The listing builds one solid part. Answer for the finished solid, in the listing's coordinates (mm). Face numbers are marked on the shaded views. Give positions to 0.01 mm unless a question says otherwise; leave off trailing zeros. Order: outer loops, then holes, each group sorted by start corner. A loop starts at its lowest first (then second) coordinate and runs counter-clockwise, first axis right, second up. Notation, with made-up numbers: (-3.5, 72) - (4.5, 72) arc R30 cw to (4.5, 103) - close; hole circle Ø1 at (5, 73). An arc over 180 degrees is marked (long way). Answer as a JSON object with one key per item and string values. Group by question number.
Q1. Given pin 1 (10 mm diameter, centred on x = 122, y = 17, fed in from -Z); pin 2 (1.5 mm diameter, centred on x = 75.5, y = 19, fed in from +Z); pin 3 (12 mm diameter, centred on x = 103, y = -7, fed in from +Z), each flat-ended and moving along its own axis, determine where each tip first touches the part or whether it passes through.
Q2. A cutting plane is placed at A-A, the plane z = -9.5. Give the vertices of the cut face in (x, y), and give its area (3 significant figures).
Q3. A cutting plane is placed at C-C, the plane x = 64. Give the vertices of the cut face in (y, z).
Q4. The mould has two halves that part along Y. Classify the marked faces 1, 2 and 3: released by +Y, released by -Y, zero draft, split by the parting line, or undercut.
Q5. A cutting plane is placed at D-D, the plane z = 49. Give the vertices of the cut face in (x, y), and give its area (3 significant figures).
Q6. Consider line 1 (Z direction, x = 0, y = -1); line 2 (X direction, y = -43, z = 0); line 3 (Y direction, x = 173, z = -2). Determine where each line is inside the solid, lowest interval first.
Q7. A cutting plane is placed at B-B, the plane y = -56.5. Give the vertices of the cut face in (x, z), and give its area (3 significant figures).
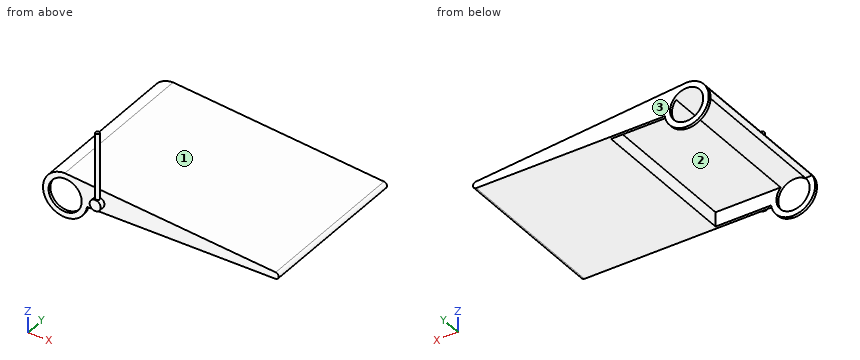
from build123d import *

# Parameters (mm, degrees)
F0_R     = 15
F1_DEPTH = 72.5
F2_W     = 140
F2_H     = 31.716244
F3_DEPTH = 70
F4_R     = 5
F5_DEPTH = 5
F6_R     = 1.75
F7_DEPTH = 70


with BuildPart() as f1:
    # F0 (on Front) → F1 (new body, symmetric)
    with BuildSketch(Plane.XZ):
        with BuildLine():
            Line((190.266781, 2.988114), (-0.258226, 19.998333))
            ThreePointArc((-0.258226, 19.998333), (-15.080984, -13.136359), (19.773847, -2.999164))
            Line((19.773847, -2.999164), (189.92918, -2.999164))
            Line((189.92918, -2.999164), (190.07082, -2.999164))
            ThreePointArc((190.07082, -2.999164), (192.998394, -0.098136), (190.266781, 2.988114))
        make_face()
        Circle(F0_R, mode=Mode.SUBTRACT)
    extrude(amount=F1_DEPTH, both=True)

    # F2 (on Right) → F3 (cut, symmetric)
    with BuildSketch(Plane.YZ):
        with Locations((0, -5.858122)):
            Rectangle(F2_W, F2_H)
    extrude(amount=F3_DEPTH, both=True, mode=Mode.SUBTRACT)

    # F4 (on face) → F5 (join)
    with BuildSketch(Plane.XZ.offset(72.5)):
        with Locations((30.506512, 5.24428)):
            Circle(F4_R)
    extrude(amount=F5_DEPTH)

    # F6 (on Top) → F7 (join)
    with BuildSketch(Plane.XY):
        with Locations((30.820567, -74.847832)):
            Circle(F6_R)
    extrude(amount=F7_DEPTH)


solid = f1.part
Reply:
{
 "1": {"pin 1": "stops at z = -3", "pin 2": "stops at z = 13.3", "pin 3": "stops at z = 11.32"},
 "2": {"outline": "(-17.6, -72.5) - (-11.61, -72.5) - (-11.61, -70) - (-17.6, -70) - close; (-17.6, 70) - (-11.61, 70) - (-11.61, 72.5) - (-17.6, 72.5) - close; (11.61, -72.5) - (17.6, -72.5) - (17.6, -70) - (11.61, -70) - close; (11.61, 70) - (17.6, 70) - (17.6, 72.5) - (11.61, 72.5) - close", "area": "59.9 mm^2"},
 "3": {"outline": "(-72.5, -3) - (-70, -3) - (-70, 10) - (70, 10) - (70, -3) - (72.5, -3) - (72.5, 14.26) - (-72.5, 14.26) - close"},
 "4": {"face 1": "zero draft", "face 2": "undercut", "face 3": "released by +Y"},
 "5": {"outline": "circle Ø3.5 at (30.82, -74.85)", "area": "9.62 mm^2"},
 "6": {"line 1": "z = 15 to 19.98", "line 2": "x = 70 to 193", "line 3": "y = -72.5 to 72.5"},
 "7": {"outline": "(-17.32, 10) - (-11.18, 10) arc R15 cw to (11.18, 10) - (70, 10) - (70, -3) - (190.07, -3) arc R3 ccw to (190.27, 2.99) - (-0.26, 20) arc R20 ccw to start", "area": "1,900 mm^2"}
}
